Part model, mm, in its own coordinate system. Coordinates: 2 decimals unless noted, no trailing zeros. Order: outer loops, then holes, each group sorted by start corner. A loop starts at its lowest first (then second) coordinate and runs counter-clockwise, first axis right, second up.
1) Cut at A-A (y = -1488). List the corners of the cut face in (x, z), and give its area (3 significant figures).
2) Pin check, flat tips, straight feed: pin 1 Ø11 at (x, y) = (30, -2160) entering from +Z; pin 2 Ø3 at (y, z) = (-471, -9) entering from -X; pin 3 Ø12 at (x, z) = (269.5, -70) entering from +Y; pin 4 Ø1 at (y, z) = (-1781, -53) entering from +X. Stop position of each tip, or through.
3) Wall check: L1, parallel to X at y = -2048, z = -32; L2, parallel to Z at x = 48.5, y = -1534.5; L3, parallel to X at y = -2160, z = -57.6. Give the ranges that are in metal, low to high.
4) Cut at B-B (x = 112). List the corners of the cut face in (y, z), and give its area (3 significant figures).
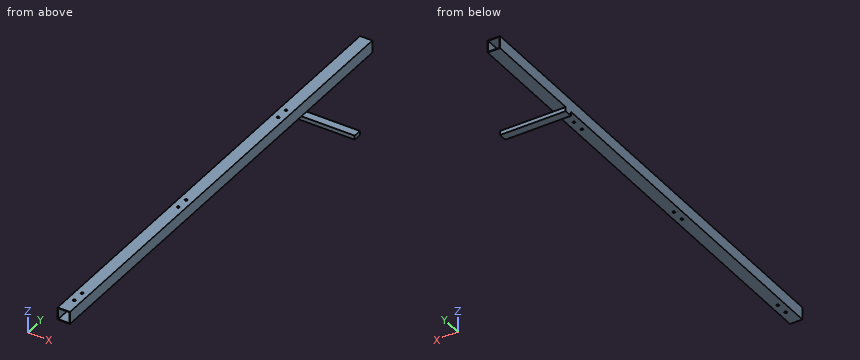
```python
from build123d import *

# Parameters (mm, degrees)
F0_W     = 60
F0_H     = 60
F0_W_2   = 54
F0_H_2   = 54
F1_DEPTH = 2300
F2_R     = 6
F3_DEPTH = 100
F4_W     = 318.082194
F4_H     = 40
F5_DEPTH = 20


with BuildPart() as f1:
    # F0 (on Front) → F1 (new body)
    with BuildSketch(Plane.XZ):
        with Locations((30, -30)):
            Rectangle(F0_W, F0_H)
        with Locations((30, -30)):
            Rectangle(F0_W_2, F0_H_2, mode=Mode.SUBTRACT)
    extrude(amount=F1_DEPTH)

    # F2 (on face) → F3 (cut)
    with BuildSketch(Plane(origin=(0, 0, -60), x_dir=(1, 0, 0), z_dir=(0, 0, -1))):
        with Locations((30, 610.001519)):
            Circle(F2_R)
        with Locations((30, 670.001519)):
            Circle(F2_R)
        with Locations((30, 1430)):
            Circle(F2_R)
        with Locations((30.426905, 1370.001519)):
            Circle(F2_R)
        with Locations((30, 2220)):
            Circle(F2_R)
        with Locations((30, 2160)):
            Circle(F2_R)
    extrude(amount=-F3_DEPTH, mode=Mode.SUBTRACT)

    # F4 (on face) → F5 (join)
    with BuildSketch(Plane(origin=(0, 0, -60), x_dir=(1, 0, 0), z_dir=(0, 0, -1))):
        with Locations((159.041097, 520)):
            Rectangle(F4_W, F4_H)
    extrude(amount=F5_DEPTH)


solid = f1.part
```
Geometry check:
1. outline: (0, -60) - (60, -60) - (60, 0) - (0, 0) - close; hole (3, -57) - (57, -57) - (57, -3) - (3, -3) - close
1. area: 684 mm2
2. pin 1: passes through
2. pin 2: stops at x = 0
2. pin 3: stops at y = -500
2. pin 4: stops at x = 60
3. L1: x = 0 to 3, 57 to 60
3. L2: z = -60 to -57, -3 to 0
3. L3: x = 0 to 24, 36 to 60
4. outline: (-540, -80) - (-500, -80) - (-500, -60) - (-540, -60) - close
4. area: 800 mm2
